Autodesk Inventor part; units mm, degrees
ref_plane "YZ Plane" through (0, 0, 0) normal (1, 0, 0) x (0, 1, 0)
ref_plane "XZ Plane" through (0, 0, 0) normal (0, 1, 0) x (-1, 0, 0)
ref_plane "XY Plane" through (0, 0, 0) normal (0, 0, 1) x (1, 0, 0)
sketch "Sketch1" plane through (0, 0, 0) normal (0, 1, 0) x (-1, 0, 0)
  line L0 (0, 0) -> (0, -41.275)
  line L1 (0, -41.275) -> (0, -36.5125)
  line L2 (0, -36.5125) -> (0, -23.4315)
  circle A0 centre (0, -36.5125) radius 1.27
  circle A1 centre (0, -23.4315) radius 1.27
  line L3 (0, -41.275) -> (3.175, -41.275)
  line L4 (3.175, -41.275) -> (3.175, 0)
  line L5 (3.175, 0) -> (0, 0)
  line L6 (0, -41.275) -> (-6.35, -41.275)
  line L7 (-6.35, -41.275) -> (-6.35, 0)
  line L8 (-6.35, 0) -> (0, 0)
  dimension "d0" = 41.275
  dimension "d1" = 4.7625
  dimension "d2" = 13.081
  dimension "d3" = 2.54
  dimension "d4" = 2.54
  dimension "d5" = 3.175
  dimension "d6" = 6.35
extrude "Extrusion1" add sketch "Sketch1" along normal blind 6.35
extrude "Extrusion2" cut sketch "Sketch1" along normal blind 6.35 contours A1 L0 | L0 A1 | A0 L0 | L0 A0
sketch "Sketch3" plane through (-3.175, 0, 0) normal (0, 0, 1) x (1, 0, 0)
  line L0 (0, 0) -> (9.525, 0)
  line L1 (9.525, 0) -> (9.525, 6.35)
  line L2 (0, 6.35) -> (9.525, 6.35)
  line L3 (0, 0) -> (0, 6.35)
  circle A0 centre (6.35, 3.175) radius 1.27
  line L4 (6.35, 3.175) -> (2.0066, 3.175)
  line L5 (2.0066, 3.175) -> (2.0066, 0)
  line L6 (9.525, 0) -> (0, 0)
  line L7 (6.35, 3.175) -> (6.35, -8.6614)
  line L8 (2.0066, 0) -> (2.0066, -8.6614)
  line L9 (2.0066, -8.6614) -> (2.0066, -10.5664)
  line L10 (2.0066, -10.5664) -> (10.2616, -10.5664)
  line L11 (10.2616, -10.5664) -> (10.2616, -8.6614)
  line L12 (10.2616, -8.6614) -> (6.35, -8.6614)
  line L13 (0, 0) -> (0, -10.5664)
  line L14 (0, -10.5664) -> (2.0066, -10.5664)
  line L15 (0, 0) -> (2.0066, 0)
  line L16 (6.35, -8.6614) -> (2.0066, -8.6614)
  line L17 (2.0066, -8.6614) -> (2.0066, 0)
  line L18 (6.35, 3.175) -> (6.35, -3.175)
  line L19 (9.525, 0) -> (2.0066, 0)
  line L20 (2.0066, 0) -> (2.0066, -3.175)
  line L21 (2.0066, -3.175) -> (9.525, -3.175)
  line L22 (9.525, -3.175) -> (9.525, 0)
  point P0 (3.175, 0)
  dimension "d11" = 2.54
  dimension "d14" = 3.175
  dimension "d15" = 9.525
  dimension "d16" = 4.3434
  dimension "d17" = 11.8364
  dimension "d18" = 1.905
  dimension "d19" = 8.255
  dimension "d22" = 6.35
extrude "Extrusion3" cut sketch "Sketch3" against normal blind 8.89 contours L7 L4 A0 | A0 L4 L7
extrude "Extrusion4" add sketch "Sketch3" against normal blind 7.62 contours L0 L8 L9 L14 L13 | L9 L16 L12 L11 L10
extrude "Extrusion5" add sketch "Sketch3" against normal blind 7.62 contours L0 L7 L21 L8 | L0 L22 L21 L7
fillet "Fillet1" radius 3.175 1 edges at (6.35, 3.175, -41.275)
fillet "Fillet2" radius 0.762 2 edges at (6.35, -3.175, -3.81) (7.0866, -8.6614, -3.81)
properties part number "photoTransistorHolderRight"
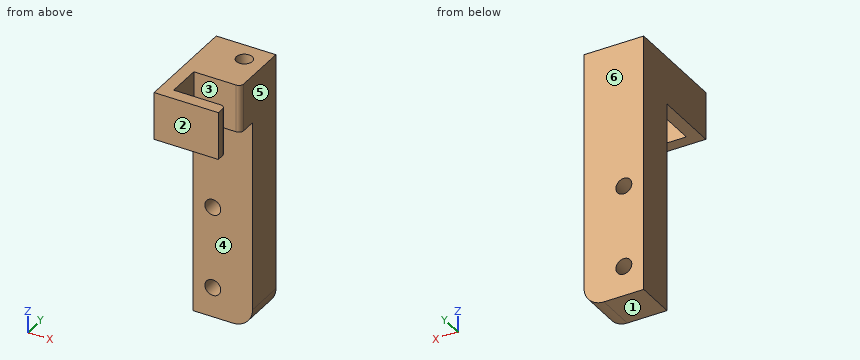
Geometry: final body of the model. Coordinates: model frame, mm. Face numbers are marked on the shaded views. A direction names the side the tool comes from. Coordinates: 2 decimals unless noted, no trailing zeros. Order: outer loops, then holes, each group sorted by start corner. A loop starts at its lowest first (then second) coordinate and runs counter-clockwise, first axis right, second up.
(1) Access query for the marked faces 4, 5 and 6. Directions: +Z, -Z, +X, -X, +Y, -Y. A direction counts if a zero-diameter tool reaches every point of the face in a straight line with its end or side. Return the directions, or none.
(2) First-contact query: pin 1 (3 mm diameter, centred on x = 3.5, y = -3.5, fed in from -Z); pin 2 (0.8 mm diameter, centred on x = 3, y = 3, fed in from +Z); pin 3 (7 mm diameter, centred on y = 0, z = -24.5, fed in from +X); pin 4 (6 mm diameter, centred on y = -6.5, z = -5.5, fed in from +X). Flat tips, straight axial feed; report the tip coordinate or a pass-through.
(3) Draft query along Y for the marked faces 1, 2 and 3. Return one class per face: pulls with the +Y half, pulls with the -Y half, needs draft (parallel to the pull), parting line crosses it, or undercut.
(4) Section query A-A (x = 0). State how many separate pieces and enclosed holes the cut face has, plus the area to 3 significant figures.
(5) Section query D-D (z = -31). Return the cut outline in (x, y) (3 decimals).
(6) Section query C-C (y = -6.5). Return the cut outline in (x, z) (3 decimals).
(7) Material intervals for probe 1 along Z at (x, y) = (0, 3) (1 decimal); probe 2 along Y at (x, z) = (3, -6) (3 decimals); probe 3 along Z at (x, y) = (-0.25, -1.75), sorted ascending.
Solution:
1. face 4: -Z, +X, -X, -Y
1. face 5: +Z, -Z, +X, +Y
1. face 6: +Z, -Z, +X, -X, +Y
2. pin 1: stops at z = -7.62
2. pin 2: stops at z = -8.89
2. pin 3: stops at x = 6.35
2. pin 4: stops at x = 7.09
3. face 1: needs draft
3. face 2: pulls with the -Y half
3. face 3: undercut
4. separate pieces: 4
4. enclosed holes: 0
4. area: 269 mm2
5. outline: (-3.175, 0) - (6.35, 0) - (6.35, 6.35) - (-3.175, 6.35) - close
6. outline: (-3.175, -7.62) - (-1.168, -7.62) - (-1.168, 0) - (-3.175, 0) - close
7. probe 1: z = -41.3 to -37.8, -35.2 to -24.7, -22.2 to 0
7. probe 2: y = -10.566 to -8.661, -3.175 to 1.917, 4.433 to 6.35
7. probe 3: z = -7.62 to 0
